For this review, take the finished solid that the model builds, in its own axes (mm). Face numbers are marked on the shaded views. A direction names the side the tool comes from. Coordinates: 2 decimals unless noted, no trailing zeros. Loops run counter-clockwise (first coordinate to the right, second up) from the corner with the lowest first, then second, coordinate; pieces in that order, holes last.
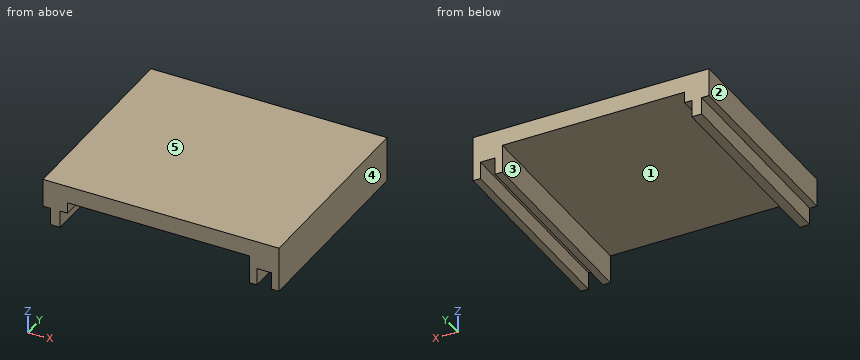
Autodesk Fusion 360 part; units mm, degrees
sketch "Sketch1" plane through (0, 22, 0) normal (0, 1, 0) x (-1, 0, 0)
  line L0 (11.5698, 0.25) -> (15.3, 0.25)
  line L1 (15.3, 0.25) -> (15.3, -0.5)
  line L2 (15.3, -0.5) -> (15.6004, -0.5)
  line L3 (15.6004, -0.5) -> (15.6004, -1.2)
  line L4 (15.6004, -1.2) -> (16.0004, -1.2)
  line L5 (16.0004, -1.2) -> (16.0004, -0.5)
  line L6 (16.0004, -0.5) -> (16.3, -0.5)
  line L7 (16.3, -0.5) -> (16.3, 1.05)
  line L8 (16.3, 1.05) -> (5, 1.05)
  line L9 (11.5698, -1.2) -> (11.5698, 0.25)
  line L10 (11.5698, -0.6208) -> (11.2698, -0.6208) construction
  line L11 (11.2698, -0.5) -> (11.2698, -1.2)
  line L12 (11.2698, -0.5) -> (10.5698, -0.5)
  line L13 (10.5698, -0.5) -> (10.5698, -1.2)
  line L14 (10.5698, -0.678) -> (10.2698, -0.678) construction
  line L15 (10.2698, 1.05) -> (10.2698, -1.2)
  line L16 (10.2698, 1.05) -> (16.3, 1.05)
  line L17 (16.3, -0.5) -> (16.0004, -0.5)
  line L18 (16.0004, -1.2) -> (15.6004, -1.2)
  line L19 (15.6004, -0.5) -> (15.3, -0.5)
  line L20 (15.3, 0.25) -> (11.5698, 0.25)
  line L21 (11.5698, -1.2) -> (11.2698, -1.2)
  line L22 (11.5698, -1.2) -> (11.2698, -1.2)
  line L23 (11.2698, -0.5) -> (10.5698, -0.5)
  line L24 (10.5698, -1.2) -> (10.2698, -1.2)
  line L25 (10.2698, 1.05) -> (16.3, 1.05)
  line L26 (16.3, -0.5) -> (16.0004, -0.5)
  line L27 (16.0004, -1.2) -> (15.6004, -1.2)
  line L28 (15.6004, -0.5) -> (15.3, -0.5)
  line L29 (15.3, 0.25) -> (11.5698, 0.25)
  dimension "d14" = 0.3
  dimension "d15" = 0.7
  dimension "d16" = 0.3
extrude "Extrude1" add sketch "Sketch1" along normal blind 8.2 makes body 1
copy_body "Body->Comp1" bodies 1 removing the originals makes body 2 in component "Component"
move_face "OffsetFaces1" offset 0.3 1 faces at (-12.8132, 24.7333, 0.25) on bodies 2 in component "Component"
move_face "OffsetFaces2" offset -0.4 1 faces at (-12.2798, 27.4667, 1.05) on bodies 2 in component "Component"
move_face "OffsetFaces3" offset 3.3 1 faces at (-10.2698, 24.7333, 0.0333) on bodies 2 in component "Component"
move_face "OffsetFaces4" offset -3.3 1 faces at (-10.5698, 24.7333, -0.7333) on bodies 2 in component "Component"
move_face "OffsetFaces5" offset 3.3 1 faces at (-11.2698, 24.7333, -0.7333) on bodies 2 in component "Component"
move_face "OffsetFaces6" offset -3.3 1 faces at (-11.5698, 27.4667, -0.8167) on bodies 2 in component "Component"
move_face "OffsetFaces7" offset -4.2 1 faces at (-10.5132, 22, 0.4167) on bodies 2 in component "Component"
move_face "OffsetFaces8" offset -0.1 1 faces at (-8.2698, 28.8667, -0.4333) on bodies 2 in component "Component"
move_face "OffsetFaces9" offset 0.1 1 faces at (-7.9698, 27.5333, -0.7333) on bodies 2 in component "Component"
move_face "OffsetFaces10" offset 4.255 1 faces at (-10.4798, 26.2, 0.4167) on bodies 2 in component "Component"
move_face "OffsetFaces11" offset 0.3 1 faces at (-6.9698, 24.6967, 0.0333) on bodies 2 in component "Component"
move_face "OffsetFaces12" offset 0.3 1 faces at (-7.8698, 24.6967, -0.7333) on bodies 2 in component "Component"
move_face "OffsetFaces13" offset -0.3 1 faces at (-7.2698, 24.6967, -0.7333) on bodies 2 in component "Component"
move_face "OffsetFaces14" offset -0.3 1 faces at (-8.1698, 24.6967, -0.8167) on bodies 2 in component "Component"
component "Component" placed x (1, 0, 0) y (0, 1, 0) z (0, 0, 1) at (0, 0, 0)
Q1. Machinability: for the marked faces 1 and 2, which of the approach directions +Z, -Z, +X, -X, +Y, -Y give a long, thin tool a straight path to every point of the face, cutting with its end or side? Answer none if there is none.
Q2. For pin 1 Ø3.5 at (x, y) = (-11.5, 27.5) entering from -Z, flat-tipped, find the tip position at first contact; note if it passes through.
Q3. Consider section B-B (y = 25.5). State the section outline as (x, z) points.
Q4. The part is to be moulded in two halves that separate along X. For the marked faces 3, 4 and 5, say which applies: +X half, -X half, draft (parallel to the pull), parting line (faces both ways), or undercut.
Q5. Consider section C-C (x = -7.25). State the section outline as (y, z) points (3 decimals).
Q6. Wall thickness on probe 1 along X at (y, z) = (28.75, -0.55); probe 2 along X at (y, z) = (28.5, -0.35); probe 3 along Z at (x, y) = (-12.25, 28): over which ranges is each line inside the solid? List them lowest first.
Q7. Consider section A-A (z = -1). State the section outline as (x, y) points (3 decimals).
Q8. Consider section D-D (x = -9.5). State the section outline as (y, z) points (3 decimals), then the cut area to 3 significant figures.
Model answer:
1. face 1: -Z, +Y, -Y
1. face 2: +Z, -Z, -X, +Y, -Y
2. pin 1: stops at z = -0.05
3. outline: (-16.3, -0.5) - (-16, -0.5) - (-16, -1.2) - (-15.6, -1.2) - (-15.6, -0.5) - (-15.3, -0.5) - (-15.3, -0.05) - (-7.87, -0.05) - (-7.87, -1.2) - (-7.57, -1.2) - (-7.57, -0.5) - (-6.97, -0.5) - (-6.97, -1.2) - (-6.67, -1.2) - (-6.67, 0.65) - (-16.3, 0.65) - close
4. face 3: undercut
4. face 4: +X half
4. face 5: draft
5. outline: (21.945, -0.5) - (30.2, -0.5) - (30.2, 0.65) - (21.945, 0.65) - close
6. probe 1: x = -16 to -15.6, -7.87 to -7.57, -6.97 to -6.67
6. probe 2: x = -16.3 to -15.3, -7.87 to -6.67
6. probe 3: z = -0.05 to 0.65
7. outline: (-16, 21.945) - (-15.6, 21.945) - (-15.6, 30.2) - (-16, 30.2) - close; (-7.87, 21.945) - (-7.57, 21.945) - (-7.57, 30.2) - (-7.87, 30.2) - close; (-6.97, 21.945) - (-6.67, 21.945) - (-6.67, 30.2) - (-6.97, 30.2) - close
8. outline: (21.945, -0.05) - (30.2, -0.05) - (30.2, 0.65) - (21.945, 0.65) - close
8. area: 5.78 mm2
